Here's how the part is built. I have some questions about the finished solid (model axes, mm). A direction names the side the tool comes from. Round coordinates to 2 decimals unless told otherwise and drop trailing zeros. Loops run counter-clockwise (first coordinate to the right, second up) from the corner with the lowest first, then second, coordinate; pieces in that order, holes last. Notation, with made-up numbers: (71.5, -19) - (128.5, -19) arc R25 ccw to (128.5, 1) - close; hole circle Ø2 at (-15, 82). An arc over 180 degrees is marked (long way). Answer as a JSON object with one key per item and string values. Group by question number.
1) I want a section at C-C, the plane z = 9.5. Please give me the cut outline in (x, y), then the cut area to 3 significant figures.
2) I want a section at A-A, the plane y = 0. Please give me the cut outline in (x, z).
3) Which directions (+Z, -Z, +X, -X, +Y, -Y) give clear straight access to the entire face, cutting with the end or side of a thin tool? Please do faces 1 (the face through (3, -3, 0)), 2 (the face through (0.1, -13.4, 2.5)), 3 (the face through (-4, 7, 16.5)).
4) Will these pins go through, and if not, where does the flat tip stop? P1, Ø1, axis at y = -2.5, z = 16.5, coming from the -X side; P2, Ø4, axis at x = -6, z = 10.5, coming from the +Y side; P3, Ø4, axis at y = -11.5, z = 16, coming from the +X side.
5) I want a section at D-D, the plane y = -12. Please give me the cut outline in (x, z), then the cut area to 3 significant figures.
6) If we mould it in two halves opening along Y, with no side actions, what happens to faces 4 (the face through (10.316, 7.91, 6.556)), 5 (the face through (-0.867, -3.905, 9.38)), 6 (the face through (3, -3, 18.5))? For each: pulls with the +Y half, pulls with the -Y half, needs draft (parallel to the pull), parting line crosses it, or undercut.
7) If I drill on line 1 along Z through (x, y) = (-11, -9); line 2 along Y through (x, z) = (0, 14.5); line 3 along Z through (x, y) = (12.25, 2.5), over which ranges is the centre line in solid material (lowest first)? Write a range as [from, to].
from build123d import *

# Parameters (mm, degrees)
SKIZZE1_R                       = 15
AUFSATZ_LINEAR_AUSTRAGEN1_DEPTH = 16.5
SCHNITT_LINEAR_AUSTRAGEN1_REACH = 28.875
SKIZZE2_R                       = 4
AUFSATZ_LINEAR_START            = 2
SKIZZE4_R                       = 7.5
SKIZZE4_R_2                     = 4
AUFSATZ_LINEAR_AUSTRAGEN2_DEPTH = 2
SKIZZE3_W                       = 2
SKIZZE3_H                       = 8


with BuildPart() as part:
    # Skizze1 → Aufsatz-Linear austragen1 (new body)
    with BuildSketch(Plane(origin=(0, 0, 0), x_dir=(0, 1, 0), z_dir=(0, 0, 1))):
        with Locations(Location((0, 0, 0), (0, 0, 270))):
            Circle(SKIZZE1_R)
    extrude(amount=AUFSATZ_LINEAR_AUSTRAGEN1_DEPTH)

    # Skizze2 → Schnitt-Linear austragen1 (cut, up to next)
    with BuildSketch(Plane.XY.offset(16.5), mode=Mode.PRIVATE) as schnitt_linear_austragen1_sk1:
        Circle(SKIZZE2_R)
    schnitt_linear_austragen1_tool1 = extrude(schnitt_linear_austragen1_sk1.sketch, amount=-SCHNITT_LINEAR_AUSTRAGEN1_REACH, mode=Mode.PRIVATE) & part.part
    add(schnitt_linear_austragen1_tool1.solids().sort_by_distance((0, 0, 16.5))[0], mode=Mode.SUBTRACT)

    # Skizze4 → Aufsatz-Linear austragen2 (add)
    with BuildSketch(Plane.XY.offset(16.5).offset(AUFSATZ_LINEAR_START)):
        Circle(SKIZZE4_R)
        Circle(SKIZZE4_R_2, mode=Mode.SUBTRACT)
    extrude(amount=-AUFSATZ_LINEAR_AUSTRAGEN2_DEPTH)

    # Skizze3 → Schnitt-Rotation1 (revolve, cut)
    with BuildSketch(Plane(origin=(0, 0, 0), x_dir=(-1, 0, 0), z_dir=(0, 1, 0)), mode=Mode.PRIVATE) as schnitt_rotation1_sk:
        with Locations((-14, 6.5)):
            Rectangle(SKIZZE3_W, SKIZZE3_H)
    revolve(schnitt_rotation1_sk.sketch.rotate(Axis((0, 0, 0), (0, 0, 1)), 180), axis=Axis((0, 0, 0), (0, 0, 1)), mode=Mode.SUBTRACT)


solid = part.part
Outcome:
{
 "1": {"outline": "circle Ø26 at (0, 0); hole circle Ø8 at (0, 0)", "area": "481 mm^2"},
 "2": {"outline": "(-15, 0) - (-4, 0) - (-4, 18.5) - (-7.5, 18.5) - (-7.5, 16.5) - (-15, 16.5) - (-15, 10.5) - (-13, 10.5) - (-13, 2.5) - (-15, 2.5) - close; (4, 0) - (15, 0) - (15, 2.5) - (13, 2.5) - (13, 10.5) - (15, 10.5) - (15, 16.5) - (7.5, 16.5) - (7.5, 18.5) - (4, 18.5) - close"},
 "3": {"face 1": "-Z, +X, -X, +Y, -Y", "face 2": "none", "face 3": "+Z"},
 "4": {"P1": "x = -14.87", "P2": "y = 14.46", "P3": "x = 11.61"},
 "5": {"outline": "(-9, 0) - (9, 0) - (9, 2.5) - (5, 2.5) - (5, 10.5) - (9, 10.5) - (9, 16.5) - (-9, 16.5) - (-9, 10.5) - (-5, 10.5) - (-5, 2.5) - (-9, 2.5) - close", "area": "233 mm^2"},
 "6": {"face 4": "parting line crosses it", "face 5": "undercut", "face 6": "needs draft"},
 "7": {"line 1": "[0, 2.5], [10.5, 16.5]", "line 2": "[-15, -4], [4, 15]", "line 3": "[0, 16.5]"}
}
